Autodesk Inventor part; units mm, degrees
ref_plane "YZ Plane" through (0, 0, 0) normal (1, 0, 0) x (0, 1, 0)
ref_plane "XZ Plane" through (0, 0, 0) normal (0, 1, 0) x (-1, 0, 0)
ref_plane "XY Plane" through (0, 0, 0) normal (0, 0, 1) x (1, 0, 0)
sketch "Sketch1" plane through (0, 0, 0) normal (0, 0, 1) x (1, 0, 0)
  circle A0 centre (0, 0) radius 10
  dimension "d0" = 20
extrude "Extrusion1" add sketch "Sketch1" along normal blind 3
sketch "Sketch2" plane through (0, 0, 3) normal (0, 0, 1) x (1, 0, 0)
  point P0 (0, 0)
  point P1 (0, 0)
hole "Hole1" at (0, 0, 3) direction (0, 0, -1) diameter 3 end through all
sketch "Sketch4" plane through (0, 0, 3) normal (0, 0, 1) x (1, 0, 0)
  circle A0 centre (0, 0) radius 10
  circle A1 centre (0, 20) radius 2.5
  circle A2 centre (0, 0) radius 1.5
  circle A3 centre (0, 0) radius 4.9374
  line L0 (-4.9006, 0.6017) -> (-2.4814, 20.3047)
  line L1 (2.4814, 20.3047) -> (4.9006, 0.6017)
  dimension "d17" = 20
  dimension "d25" = 5
  dimension "d26" = 20
  dimension "d28" = 14
extrude "Extrusion2" add sketch "Sketch4" against normal up to surface (3 mm away) contours L1 A3 L0 A0 | A0 L0 A1 L1 | A1 picked at (-0.6528, 8.2479)
pattern_circular "Circular Pattern1" count 5 over 360 about axis through (0, 0, -10) along (0, 0, 1) of "Extrusion2"
properties part number "Selection_Gear 1" material "Nylon 6/6"
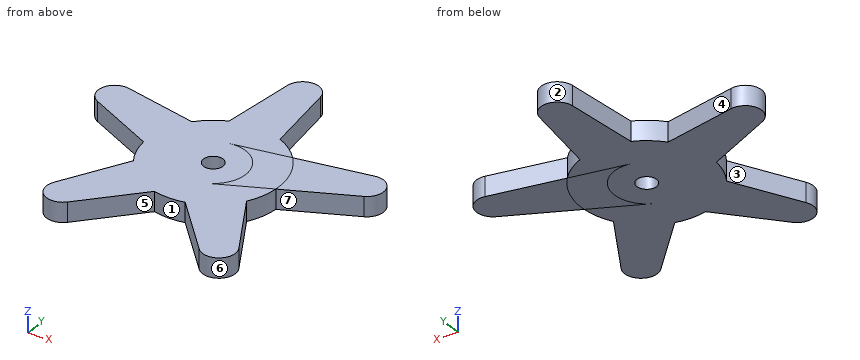
Here's how the part is built. I have some questions about the finished solid (model axes, mm). Face numbers are marked on the shaded views. A direction names the side the tool comes from. Round coordinates to 2 decimals unless told otherwise and drop trailing zeros. Order: outer loops, then holes, each group sorted by start corner. A loop starts at its lowest first (then second) coordinate and runs counter-clockwise, first axis right, second up. Notation, with made-up numbers: M 9,-24 L 56,-24 A15 cw 56,-8 Z; hole C 44.25,69 d11. An arc over 180 degrees is marked long. Return JSON: item names as keys, results as strings. Group by question number.
1. If we section it at D-D on y = -9: List the corners of the cut face in (x, z) for me.
2. If we section it at B-B on y = 0.5: List the corners of the cut face in (x, z) for me, then the cut area to 3 significant figures.
3. If we mould it in two halves opening along Y, with no side actions, what happens to the marked faces 1, 2 and 3? For each: pulls with the +Y half, pulls with the -Y half, needs draft (parallel to the pull), parting line crosses it, or undercut.
4. I'm going to push a flat-ended pin straight in: pin 1 Ø1.8 at (x, y) = (0, 0) entering from -Z. Where does the tip first touch, or does it pass through?
5. If we section it at A-A on x = 0: List the corners of the cut face in (y, z) for me.
6. Please list where these lines run through material, in increasing order: probe 1 along Y at (x, z) = (0, 2.2); probe 2 along X at (y, z) = (-12, 0.45); probe 3 along X at (y, z) = (-1, 0.3).
7. If we section it at C-C on z = 0.8: List the corners of the cut face in (x, y) for me, then the cut area to 3 significant figures.
8. On a 3-axis mill with a long thin cutter (end or side, diameter ignored), from which of +Z, -Z, +X, -X, +Y, -Y can I reach the whole of each face in a straight line? I mean the marked faces 4, 5, 6 and 7. Say none if no direction works.
Reply:
{
 "1": {"outline": "M -10.63,0 L 10.63,0 L 10.63,3 L -10.63,3 Z"},
 "2": {"outline": "M -12.76,0 L -1.41,0 L -1.41,3 L -12.76,3 Z; M 1.41,0 L 12.76,0 L 12.76,3 L 1.41,3 Z", "area": "68.0 mm^2"},
 "3": {"face 1": "pulls with the -Y half", "face 2": "pulls with the +Y half", "face 3": "undercut"},
 "4": {"pin 1": "through"},
 "5": {"outline": "M -10,0 L -1.5,0 L -1.5,3 L -10,3 Z; M 1.5,0 L 22.5,0 L 22.5,3 L 1.5,3 Z"},
 "6": {"probe 1": "-10 to -1.5, 1.5 to 22.5", "probe 2": "-12.3 to -4.44, 4.44 to 12.3", "probe 3": "-9.95 to -1.12, 1.12 to 9.95"},
 "7": {"outline": "M -20.08,3.91 L -9.97,-0.8 A10 ccw -8.53,-5.21 L -13.94,-14.97 A2.5 ccw -9.93,-17.89 L -2.32,-9.73 A10 ccw 2.32,-9.73 L 9.93,-17.89 A2.5 ccw 13.94,-14.97 L 8.53,-5.21 A10 ccw 9.97,-0.8 L 20.08,3.91 A2.5 ccw 18.54,8.63 L 7.59,6.51 A10 ccw 3.84,9.23 L 2.48,20.3 A2.5 ccw -2.48,20.3 L -3.84,9.23 A10 ccw -7.59,6.51 L -18.54,8.63 A2.5 ccw Z; hole C 0,0 d3", "area": "679 mm^2"},
 "8": {"face 4": "+Z, -Z, +Y", "face 5": "+Z, -Z, -Y", "face 6": "+Z, -Z", "face 7": "+Z, -Z, +X"}
}
